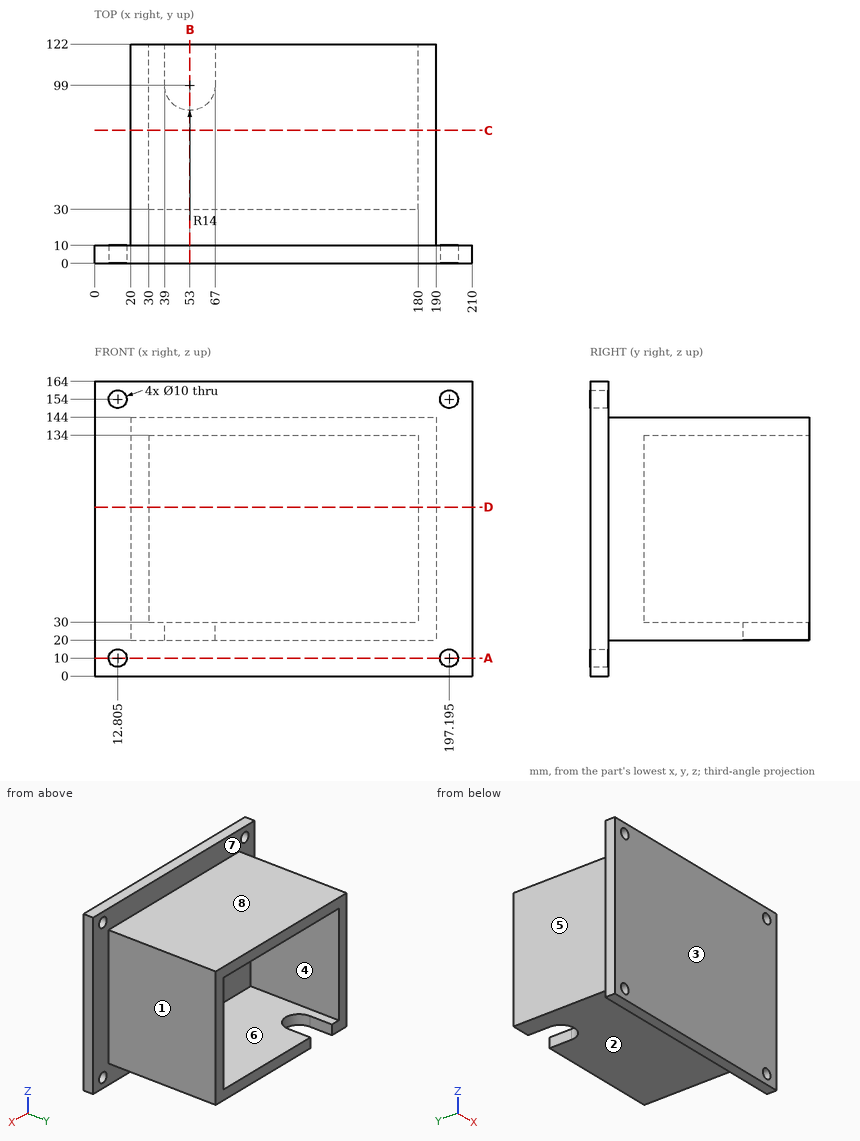
Verification items for this drawing (mm, ordinates from the low corner). A direction names the side the tool comes from. Round coordinates to 2 decimals unless told otherwise and drop trailing zeros. Loops run counter-clockwise (first coordinate to the right, second up) from the corner with the lowest first, then second, coordinate; pieces in that order, holes last. Notation, with made-up numbers: M 29.25,-9.75 L 55.25,-9.75 A14 cw 55.25,5.25 Z; hole C 11.5,83 d11. An arc over 180 degrees is marked long. Answer as a JSON object with one key per item and string values.
1. Section check A-A (z = 10). Record the boundary of the cut face in (x, y) (3 decimals).
Reply:
{"outline": "M 0,0 L 7.805,0 L 7.805,10 L 0,10 Z; M 17.805,0 L 192.195,0 L 192.195,10 L 17.805,10 Z; M 202.195,0 L 210,0 L 210,10 L 202.195,10 Z"}
2. Gauge pin test, flat ends, axial feed: P1, Ø8, axis at y = 112, z = 25.5, coming from the -X side; P2, Ø5, axis at x = 154.5, y = 95, coming from the -Z side; P3, Ø5, axis at x = 118, y = 88.5, coming from the +Z side; P4, Ø6, axis at x = 12.8, z = 10, coming from the -Y side (3 decimals). Record the tip position at first contact, or that the pin passes through.
Reply:
{"P1": "stops at x = 20", "P2": "stops at z = 20", "P3": "stops at z = 144", "P4": "passes through"}
3. Scan lines: line 1 (X direction, y = 2, z = 10) (3 decimals); line 2 (Z direction, x = 170, y = 64); line 3 (X direction, y = 93.5, z = 83). Record each from-to range of solid material in increasing order.
Reply:
{"line 1": "x = 0 to 7.805, 17.805 to 192.195, 202.195 to 210", "line 2": "z = 20 to 30, 134 to 144", "line 3": "x = 20 to 30, 180 to 190"}
4. Section check B-B (x = 53). Record the boundary of the cut face in (y, z).
Reply:
{"outline": "M 0,0 L 10,0 L 10,20 L 85,20 L 85,30 L 30,30 L 30,134 L 122,134 L 122,144 L 10,144 L 10,164 L 0,164 Z"}
5. Mould release check, pull along Z, two halves, no side actions. Record for the marked faces 6, 7 and 8: pulls with the +Z half, pulls with the -Z half, needs draft (parallel to the pull), parting line crosses it, or undercut.
Reply:
{"face 6": "undercut", "face 7": "needs draft", "face 8": "pulls with the +Z half"}
6. Section check C-C (y = 74). Record the boundary of the cut face in (x, z).
Reply:
{"outline": "M 20,20 L 190,20 L 190,144 L 20,144 Z; hole M 30,30 L 180,30 L 180,134 L 30,134 Z"}
7. Section check D-D (z = 94). Record the boundary of the cut face in (x, y), plus the area to 3 significant figures.
Reply:
{"outline": "M 0,0 L 210,0 L 210,10 L 190,10 L 190,122 L 180,122 L 180,30 L 30,30 L 30,122 L 20,122 L 20,10 L 0,10 Z", "area": "7,340 mm²"}
8. Access from +Z, -Z, +X, -X, +Y, -Y to the whole of each face (thin tool, end or side, straight path). Record for the marked faces 1, 2, 3, 4 and 5.
Reply:
{"face 1": "+Z, -Z, +X, +Y", "face 2": "-Z, +X, -X, +Y", "face 3": "+Z, -Z, +X, -X, -Y", "face 4": "+Y", "face 5": "+Z, -Z, -X, +Y"}
